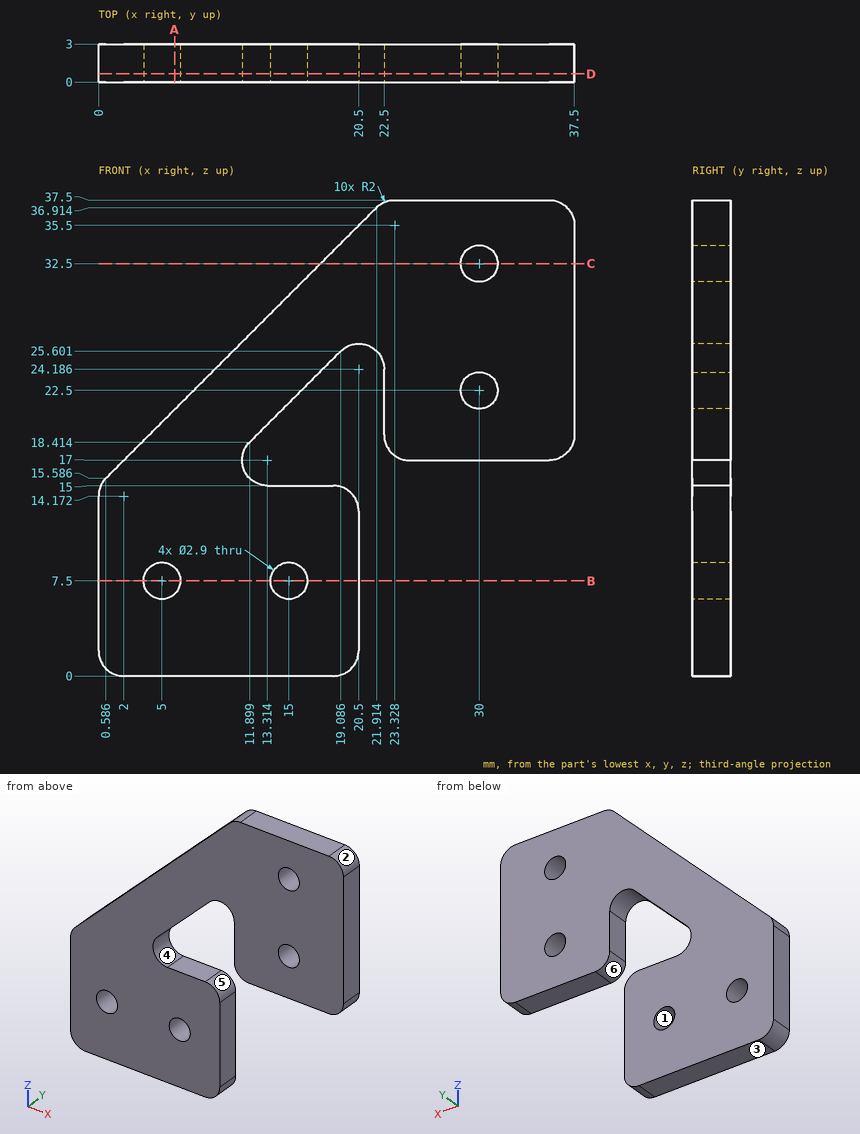
Geometry check sheet. Reference: drawing and pictorial views, mm from the part's lowest x, y, z. A direction names the side the tool comes from. Give positions to 0.01 mm unless a question says otherwise; leave off trailing zeros. Loops run counter-clockwise (first coordinate to the right, second up) from the corner with the lowest first, then second, coordinate; pieces in that order, holes last.
1. Go/stop test with flat-tipped pins: pin 1 Ø1.5 at (y, z) = (2, 6.5) entering from +X; pin 2 Ø1.5 at (y, z) = (1, 22) entering from -X. Record where each tip stops, or that it passes through.
2. Section check D-D, the plane y = 0.65. Count the separate pieces of the cut face and the enclosed holes in it, then the cut area to 3 significant figures.
3. Section check A-A, the plane x = 6. Enter the section's corners in (y, z), then the cut area to 3 significant figures.
4. Mould release check, pull along X, two halves, no side actions. Record for the marked faces 1, 2 and 3: released by +X, released by -X, zero draft, split by the parting line, or undercut.
5. Set-up check for the marked faces 4, 5 and 6: record each of +Z, -Z, +X, -X, +Y, -Y from which the full face is reachable in a straight line by a thin tool's end or side.
6. Section check C-C, the plane z = 32.5. Enter the section's corners in (x, y).
7. Thickness scan on line 1 (X direction, y = 2.2, z = 7.5); line 2 (X direction, y = 1.9, z = 8.5); line 3 (Z direction, x = 33, y = 2). Record the ranges inside material, lowest first.
8. Section check B-B, the plane z = 7.5. Enter the section's corners in (x, y).
Geometry says:
1. pin 1: stops at x = 20.5
1. pin 2: stops at x = 6.25
2. separate pieces: 1
2. enclosed holes: 4
2. area: 748 mm2
3. outline: (0, 0) - (3, 0) - (3, 6.45) - (0, 6.45) - close; (0, 8.55) - (3, 8.55) - (3, 21) - (0, 21) - close
3. area: 56.7 mm2
4. face 1: undercut
4. face 2: released by +X
4. face 3: zero draft
5. face 4: +Y, -Y
5. face 5: +X, +Y, -Y
5. face 6: -Z, +Y, -Y
6. outline: (17.5, 0) - (28.55, 0) - (28.55, 3) - (17.5, 3) - close; (31.45, 0) - (37.5, 0) - (37.5, 3) - (31.45, 3) - close
7. line 1: x = 0 to 3.55, 6.45 to 13.55, 16.45 to 20.5
7. line 2: x = 0 to 3.95, 6.05 to 13.95, 16.05 to 20.5
7. line 3: z = 17 to 37.5
8. outline: (0, 0) - (3.55, 0) - (3.55, 3) - (0, 3) - close; (6.45, 0) - (13.55, 0) - (13.55, 3) - (6.45, 3) - close; (16.45, 0) - (20.5, 0) - (20.5, 3) - (16.45, 3) - close
